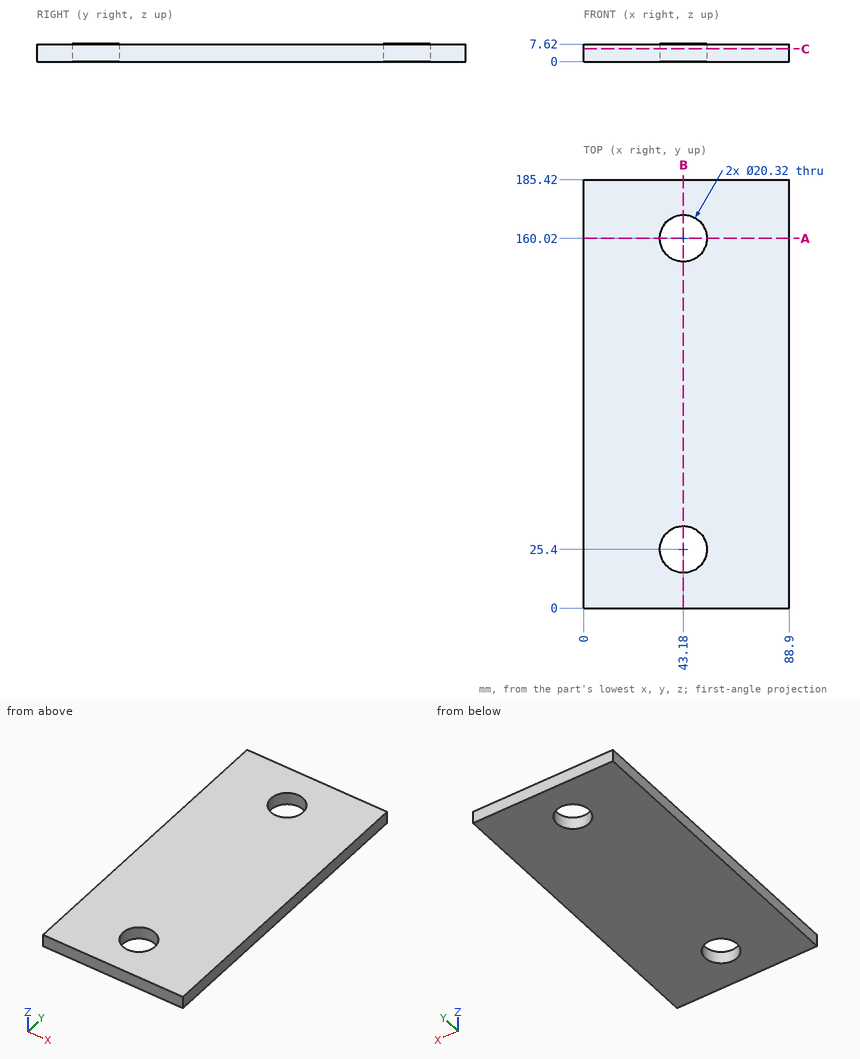
Could you check a few things on this drawing? It's one solid part, dimensions in mm from its lowest x, y, z. Round coordinates to 2 decimals unless told otherwise and drop trailing zeros. Write each loop counter-clockwise with the first axis right and the second up, starting at its lowest first coordinate (ties: lowest second). Pieces come first, ordered by that corner, then holes. Notation, with made-up numbers: (64, -25.5) -> (119, -25.5) arc R14 ccw to (119, -3.5) -> close; hole circle Ø11 at (-2.75, 26). An arc over 180 degrees is marked (long way). One line per item, written item: value.
1) Suppose I cut it at A-A on y = 160.02. List the corners of the cut face in (x, z) for me.
Filled sheet:
outline: (0, 0) -> (33.02, 0) -> (33.02, 7.62) -> (0, 7.62) -> close; (53.34, 0) -> (88.9, 0) -> (88.9, 7.62) -> (53.34, 7.62) -> close
2) Suppose I cut it at B-B on x = 43.18. List the corners of the cut face in (y, z) for me, plus the area to 3 significant figures.
Filled sheet:
outline: (0, 0) -> (15.24, 0) -> (15.24, 7.62) -> (0, 7.62) -> close; (35.56, 0) -> (149.86, 0) -> (149.86, 7.62) -> (35.56, 7.62) -> close; (170.18, 0) -> (185.42, 0) -> (185.42, 7.62) -> (170.18, 7.62) -> close
area: 1,100 mm2
3) If I drill on line 1 (Y direction, x = 43.18, z = 3); line 2 (Y direction, x = 34, z = 5); line 3 (X direction, y = 23, z = 1.5), over which ranges is the centre line in solid material (lowest first)? Write a range as [from, to].
Filled sheet:
line 1: y = [0, 15.24], [35.56, 149.86], [170.18, 185.42]
line 2: y = [0, 21.05], [29.75, 155.67], [164.37, 185.42]
line 3: x = [0, 33.31], [53.05, 88.9]
4) Suppose I cut it at C-C on z = 5.5. List the corners of the cut face in (x, y) for me, plus the area to 3 significant figures.
Filled sheet:
outline: (0, 0) -> (88.9, 0) -> (88.9, 185.42) -> (0, 185.42) -> close; hole circle Ø20.32 at (43.18, 25.4); hole circle Ø20.32 at (43.18, 160.02)
area: 15,800 mm2
